from build123d import *

# Parameters (mm, degrees)
F1_DEPTH = 38.1
F3_DEPTH = 38.1


with BuildPart() as f1:
    # F0 (on Front) → F1 (new body)
    with BuildSketch(Plane.XZ):
        Polygon((-64.931455, 8.465862), (11.268545, 8.465862), (11.268545, 18.554664), (49.368545, 18.554664), (11.268545, 46.565862), (-64.931455, 46.565862), align=None)
    extrude(amount=F1_DEPTH)

    # F2 (on face) → F3 (cut)
    with BuildSketch(Plane.XY.offset(46.565862)):
        Polygon((-39.531455, -21.6916), (-26.831455, -21.6916), (-14.131455, -21.6916), (-14.131455, -16.4084), (-39.531455, -16.4084), align=None)
    extrude(amount=-F3_DEPTH, mode=Mode.SUBTRACT)


solid = f1.part
Work out the finished part from the listing and answer in its coordinate system (mm). A direction names the side the tool comes from. Give positions to 0.01 mm unless a question says otherwise; leave off trailing zeros. Loops run counter-clockwise (first coordinate to the right, second up) from the corner with the lowest first, then second, coordinate; pieces in that order, holes last. Notation, with made-up numbers: (-18.5, 13) - (-5.5, 13) arc R18 ccw to (-5.5, 24) - close; hole circle Ø3 at (-16, 7.5). An arc over 180 degrees is marked (long way). Answer in a Markdown table with one row per item. Add a question column.
Q1. The part is cut by section B-B (z = 11). Determine the outline of the cut face in (x, y).
Q2. A tool of negligible diameter and unlimited length cuts with its end or side. For faces 1 (the flat face through (-14.131, -19, 28)), 2 (the flat face through (30.59, -18.78, 32.36)), 3 (the flat face through (11.269, -19, 13)), from which of +Z, -Z, +X, -X, +Y, -Y can it reach the whole face along a straight path? Write none if from no direction.
Q3. The part is cut by section A-A (x = -23.5). Determine the outline of the cut face in (y, z).
Q4. Consider line 1 along X through (y, z) = (-21, 13); line 2 along Y through (x, z) = (-21.5, 23); line 3 along X through (y, z) = (-3, 15). Determine where each line is inside the solid, lowest interval first.
Q5. The part is cut by section C-C (y = -25). Determine the outline of the cut face in (x, z), and give its area (3 significant figures).
Q6. Determine the mould class of faces 4 (the flat face through (-64.931, -19, 28)), 5 (the flat face through (-39.531, -19, 28)), 6 (the flat face through (-27, -16.408, 28)), 7 (the flat face through (30, -19, 18.555)) for opening direction X: released by +X, released by -X, zero draft, split by the parting line, or undercut.
Q7. Each of these flat-tipped pins is pushed along its axis until it touches: P1, Ø12, axis at x = 23, y = -33.5, coming from the -Z side; P2, Ø2.5, axis at y = -20, z = 27.5, coming from the +X side; P3, Ø3, axis at y = -25, z = 11.5, coming from the +X side. Where does it stop, or does it pass through?
Q8. The part is cut by section D-D (z = 42.5). Determine the outline of the cut face in (x, y).
Solution:
| question | item | result |
|---|---|---|
| 1 | outline | (-64.93, -38.1) - (11.27, -38.1) - (11.27, 0) - (-64.93, 0) - close; hole (-39.53, -21.69) - (-14.13, -21.69) - (-14.13, -16.41) - (-39.53, -16.41) - close |
| 2 | face 1 | +Z, -Z |
| 2 | face 2 | +Z, +X, +Y, -Y |
| 2 | face 3 | -Z, +X, +Y, -Y |
| 3 | outline | (-38.1, 8.47) - (-21.69, 8.47) - (-21.69, 46.57) - (-38.1, 46.57) - close; (-16.41, 8.47) - (0, 8.47) - (0, 46.57) - (-16.41, 46.57) - close |
| 4 | line 1 | x = -64.93 to -39.53, -14.13 to 11.27 |
| 4 | line 2 | y = -38.1 to -21.69, -16.41 to 0 |
| 4 | line 3 | x = -64.93 to 11.27 |
| 5 | outline | (-64.93, 8.47) - (11.27, 8.47) - (11.27, 18.55) - (49.37, 18.55) - (11.27, 46.57) - (-64.93, 46.57) - close |
| 5 | area | 3,440 mm² |
| 6 | face 4 | released by -X |
| 6 | face 5 | undercut |
| 6 | face 6 | undercut |
| 6 | face 7 | zero draft |
| 7 | P1 | stops at z = 18.55 |
| 7 | P2 | stops at x = 38.9 |
| 7 | P3 | stops at x = 11.27 |
| 8 | outline | (-64.93, -38.1) - (16.8, -38.1) - (16.8, 0) - (-64.93, 0) - close; hole (-39.53, -21.69) - (-14.13, -21.69) - (-14.13, -16.41) - (-39.53, -16.41) - close |
